For this review, take the finished solid that the model builds, in its own axes (mm). Round coordinates to 2 decimals unless told otherwise and drop trailing zeros. Write each loop counter-clockwise with the first axis right and the second up, starting at its lowest first coordinate (ties: lowest second). Pieces come first, ordered by that corner, then holes. Notation, with made-up numbers: (31, 30.5) -> (66, 30.5) arc R20 cw to (66, 41.5) -> close; hole circle Ø9 at (-38, 72.5). An arc over 180 degrees is marked (long way). Answer as CSV lines item,"result". Start each with the question number.
Item 1: For pin 1 Ø1 at (y, z) = (-1, 27.5) entering from -X; pin 2 Ø1 at (x, y) = (-592, -0.5) entering from +Z; pin 3 Ø1 at (x, y) = (-349, -1) entering from +Z, all flat-tipped, find the tip position at first contact; note any pin that passes through.
Item 2: Take a section at B-B on y = -1.6. Give the boundary of the cut face in (x, z).
Item 3: Take a section at A-A on x = 0. Give the boundary of the cut face in (y, z), then the cut area to 3 significant figures.
Item 4: Wall thickness on probe 1 along Z at (x, y) = (0, -1.5); probe 2 along X at (y, z) = (-0.5, 9.5); probe 3 along Z at (x, y) = (-351, -0.2): over which ranges is each line inside the solid? List them lowest first. Write a range as from..to.
```python
from build123d import *

# Parameters (mm, degrees)
F0_R     = 14
F1_DEPTH = 2


with BuildPart() as f1:
    # F0 (on Front) → F1 (new body)
    with BuildSketch(Plane.XZ):
        with BuildLine():
            Line((-597.5, -39), (597.5, -39))
            Line((597.5, -39), (597.5, 9))
            Line((597.5, 9), (579.5, 9))
            Line((579.5, 9), (579.5, 39))
            Line((579.5, 39), (278.5, 39))
            ThreePointArc((278.5, 39), (271.470563, 22.029437), (254.5, 15))
            Line((254.5, 15), (222.5, 15))
            ThreePointArc((222.5, 15), (205.529437, 22.029437), (198.5, 39))
            Line((198.5, 39), (-316.5, 39))
            ThreePointArc((-316.5, 39), (-323.529437, 22.029437), (-340.5, 15))
            Line((-340.5, 15), (-372.5, 15))
            ThreePointArc((-372.5, 15), (-389.470563, 22.029437), (-396.5, 39))
            Line((-396.5, 39), (-579.5, 39))
            Line((-579.5, 39), (-579.5, 9))
            Line((-579.5, 9), (-597.5, 9))
            Line((-597.5, 9), (-597.5, -39))
        make_face()
        with Locations((0, 9)):
            Circle(F0_R, mode=Mode.SUBTRACT)
    extrude(amount=F1_DEPTH)


solid = f1.part
```
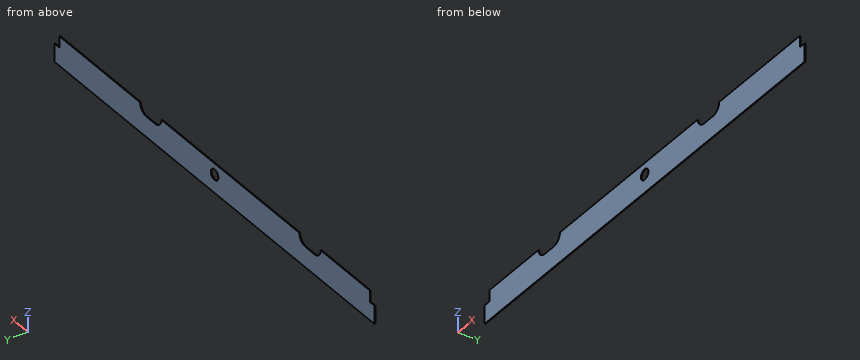
Output values:
1,pin 1,"stops at x = -579.5"
1,pin 2,"stops at z = 9"
1,pin 3,"stops at z = 15"
2,outline,"(-597.5, -39) -> (597.5, -39) -> (597.5, 9) -> (579.5, 9) -> (579.5, 39) -> (278.5, 39) arc R24 cw to (254.5, 15) -> (222.5, 15) arc R24 cw to (198.5, 39) -> (-316.5, 39) arc R24 cw to (-340.5, 15) -> (-372.5, 15) arc R24 cw to (-396.5, 39) -> (-579.5, 39) -> (-579.5, 9) -> (-597.5, 9) -> close; hole circle Ø28 at (0, 9)"
3,outline,"(-2, -39) -> (0, -39) -> (0, -5) -> (-2, -5) -> close; (-2, 23) -> (0, 23) -> (0, 39) -> (-2, 39) -> close"
3,area,"100 mm^2"
4,probe 1,"z = -39..-5, 23..39"
4,probe 2,"x = -579.5..-13.99, 13.99..579.5"
4,probe 3,"z = -39..15"
